from build123d import *

# Parameters (mm, degrees)
BOSS_EXTRUDE1_DEPTH = 0.762


with BuildPart() as part:
    # Sketch1 → Boss-Extrude1 (new body)
    with BuildSketch(Plane.XY):
        with BuildLine():
            Line((0, -76.2), (0, -9.525))
            ThreePointArc((0, -9.525), (2.789807909, -2.789807909), (9.525, 0))
            Line((9.525, 0), (76.2, 0))
            Line((76.2, 0), (76.2, -19.05))
            Line((76.2, -19.05), (19.05, -76.2))
            Line((19.05, -76.2), (0, -76.2))
        make_face()
        with BuildLine():
            Line((56.9976, -8.001), (69.6976, -8.001))
            ThreePointArc((69.6976, -8.001), (71.2216, -9.525), (69.6976, -11.049))
            Line((69.6976, -11.049), (56.9976, -11.049))
            ThreePointArc((56.9976, -11.049), (55.4736, -9.525), (56.9976, -8.001))
        make_face(mode=Mode.SUBTRACT)
        with BuildLine():
            Line((8.001, -56.9976), (8.001, -69.6976))
            ThreePointArc((8.001, -69.6976), (9.525, -71.2216), (11.049, -69.6976))
            Line((11.049, -69.6976), (11.049, -56.9976))
            ThreePointArc((11.049, -56.9976), (9.525, -55.4736), (8.001, -56.9976))
        make_face(mode=Mode.SUBTRACT)
        with BuildLine():
            Line((29.0576, -11.049), (16.3576, -11.049))
            ThreePointArc((16.3576, -11.049), (14.8336, -9.525), (16.3576, -8.001))
            Line((16.3576, -8.001), (29.0576, -8.001))
            ThreePointArc((29.0576, -8.001), (30.5816, -9.525), (29.0576, -11.049))
        make_face(mode=Mode.SUBTRACT)
        with BuildLine():
            Line((11.049, -29.0576), (11.049, -16.3576))
            ThreePointArc((11.049, -16.3576), (9.525, -14.8336), (8.001, -16.3576))
            Line((8.001, -16.3576), (8.001, -29.0576))
            ThreePointArc((8.001, -29.0576), (9.525, -30.5816), (11.049, -29.0576))
        make_face(mode=Mode.SUBTRACT)
    extrude(amount=BOSS_EXTRUDE1_DEPTH)


solid = part.part
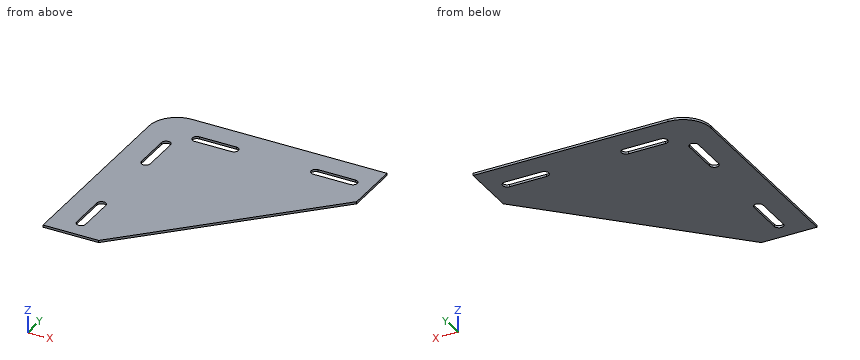
Geometry check sheet. Reference: the model listing, model coordinates, mm. Round coordinates to 2 decimals unless told otherwise and drop trailing zeros. Write each loop counter-clockwise with the first axis right and the second up, starting at its lowest first coordinate (ties: lowest second). Pieces come first, ordered by that corner, then holes. Notation, with made-up numbers: (-39, 72.25) - (-10, 72.25) arc R29 ccw to (-10, 99.25) - close; hole circle Ø1 at (80.5, 18). An arc over 180 degrees is marked (long way). One line per item, written item: value.
1. Cross-section at D-D on x = 36. Record the boundary of the cut face in (y, z).
The answers:
outline: (-59.25, 0) - (0, 0) - (0, 0.76) - (-59.25, 0.76) - close
2. Cross-section at A-A on y = -58.5. Record the boundary of the cut face in (x, z).
The answers:
outline: (0, 0) - (8, 0) - (8, 0.76) - (0, 0.76) - close; (11.05, 0) - (36.75, 0) - (36.75, 0.76) - (11.05, 0.76) - close
3. Cross-section at C-C on z = 0.45. Record the boundary of the cut face in (x, y) (3 decimals), and give its area (3 significant figures).
The answers:
outline: (0, -76.2) - (19.05, -76.2) - (76.2, -19.05) - (76.2, 0) - (9.525, 0) arc R9.525 ccw to (0, -9.525) - close; hole (8.001, -69.698) arc R1.524 ccw to (11.049, -69.698) - (11.049, -56.998) arc R1.524 ccw to (8.001, -56.998) - close; hole (8.001, -29.058) arc R1.524 ccw to (11.049, -29.058) - (11.049, -16.358) arc R1.524 ccw to (8.001, -16.358) - close; hole (16.358, -11.049) - (29.058, -11.049) arc R1.524 ccw to (29.058, -8.001) - (16.358, -8.001) arc R1.524 ccw to start; hole (56.998, -11.049) - (69.698, -11.049) arc R1.524 ccw to (69.698, -8.001) - (56.998, -8.001) arc R1.524 ccw to start
area: 3,970 mm^2
4. Scan lines: L1, parallel to X at y = -9.5, z = 0.7; L2, parallel to X at y = -19, z = 0.7; L3, parallel to Y at x = 16.5, z = 0.1. Record each from-to range of solid material in increasing order.
The answers:
L1: x = 0 to 14.83, 30.58 to 55.47, 71.22 to 76.2
L2: x = 0 to 8, 11.05 to 76.2
L3: y = -76.2 to -11.05, -8 to 0
5. Cross-section at B-B on x = 24. Record the boundary of the cut face in (y, z), and give its area (3 significant figures).
The answers:
outline: (-71.25, 0) - (-11.05, 0) - (-11.05, 0.76) - (-71.25, 0.76) - close; (-8, 0) - (0, 0) - (0, 0.76) - (-8, 0.76) - close
area: 52.0 mm^2
